Can you work these out from the model? Positions are in its coordinate system, mm. Face numbers are marked on the shaded views. A direction names the side the tool comes from. Give positions to 0.01 mm unless a question says otherwise; leave off trailing zeros. Loops run counter-clockwise (first coordinate to the right, second up) from the corner with the lowest first, then second, coordinate; pieces in that order, holes last. Notation, with made-up numbers: (84, 81.5) -> (139, 81.5) arc R32 ccw to (139, 107.5) -> close; hole circle Ø7 at (1.25, 34). An arc over 180 degrees is marked (long way). One line per question, with ' | ' between items.
from build123d import *

# Parameters (mm, degrees)
F0_R          = 12.7
F1_DEPTH      = 17.78
F2_R          = 38.1
F3_DEPTH      = 10.16
F4_R          = 12.954
F5_DEPTH      = 17.781
F5_DEPTH_BACK = 115
F6_W          = 5.08
F6_H          = 30.48
F7_DEPTH      = 38.101
F7_DEPTH_BACK = 38.101
F8_W          = 40.513
F8_H          = 5.08
F9_DEPTH      = 38.101
F9_DEPTH_BACK = 38.101
F11_DEPTH     = 6.35


# Not quite as in the source:
# - an extrude ends at something that could not be found from the text; its depth is read off the source's solid


with BuildPart() as f1:
    # F0 (on Front) → F1 (new body)
    with BuildSketch(Plane.XZ):
        Circle(F0_R)
    extrude(amount=F1_DEPTH)

    # F2 (on Front) → F3 (join)
    with BuildSketch(Plane.XZ):
        Circle(F2_R)
    extrude(amount=F3_DEPTH)

    # F4 (on Front) → F5 (cut, two sides)
    with BuildSketch(Plane.XZ) as f5_sk:
        Circle(F4_R)
    extrude(amount=F5_DEPTH, mode=Mode.SUBTRACT)
    extrude(f5_sk.sketch, amount=-F5_DEPTH_BACK, mode=Mode.SUBTRACT)

    # F6 (on Right) → F7 (cut, two sides)
    with BuildSketch(Plane.YZ) as f7_sk:
        with Locations((-2.54, 0)):
            Rectangle(F6_W, F6_H)
    extrude(amount=F7_DEPTH, mode=Mode.SUBTRACT)
    extrude(f7_sk.sketch, amount=-F7_DEPTH_BACK, mode=Mode.SUBTRACT)

    # F8 (on Top) → F9 (cut, two sides)
    with BuildSketch(Plane.XY) as f9_sk:
        with Locations((0, -2.54)):
            Rectangle(F8_W, F8_H)
    extrude(amount=-F9_DEPTH, mode=Mode.SUBTRACT)
    extrude(f9_sk.sketch, amount=F9_DEPTH_BACK, mode=Mode.SUBTRACT)

    # F10 (on face) → F11 (cut)
    with BuildSketch(Plane(origin=(0, 0, 0), x_dir=(-1, 0, 0), z_dir=(0, 1, 0))):
        with BuildLine():
            Line((1.27, -1.27), (38.0788274504, -1.27))
            ThreePointArc((38.0788274504, -1.27), (38.1, 0), (38.0788274504, 1.27))
            Line((38.0788274504, 1.27), (1.27, 1.27))
            Line((1.27, 1.27), (1.27, 38.0788274504))
            ThreePointArc((1.27, 38.0788274504), (0, 38.1), (-1.27, 38.0788274504))
            Line((-1.27, 38.0788274504), (-1.27, 1.27))
            Line((-1.27, 1.27), (-38.0788274504, 1.27))
            ThreePointArc((-38.0788274504, 1.27), (-38.1, 0), (-38.0788274504, -1.27))
            Line((-38.0788274504, -1.27), (-1.27, -1.27))
            Line((-1.27, -1.27), (-1.27, -38.0788274504))
            ThreePointArc((-1.27, -38.0788274504), (0, -38.1), (1.27, -38.0788274504))
            Line((1.27, -38.0788274504), (1.27, -1.27))
        make_face()
    extrude(amount=-F11_DEPTH, mode=Mode.SUBTRACT)


solid = f1.part
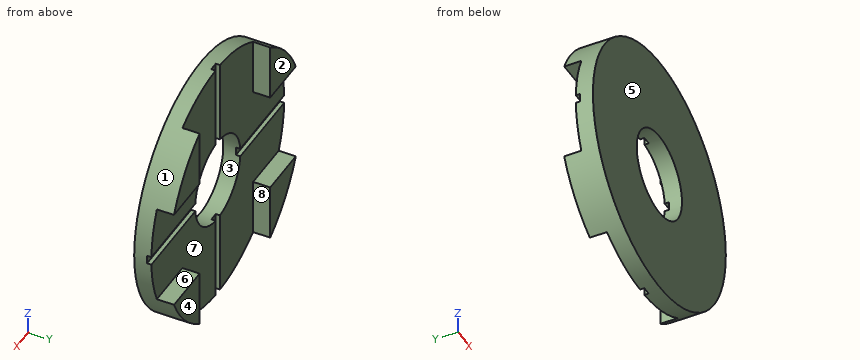
Q1. If we section it at A-A (z = 0): Write out the boundary of the cut face in (x, y).
Entries:
outline: (-38.1, -10.16) -> (-12.95, -10.16) -> (-12.95, -6.35) -> (-38.1, -6.35) -> close; (12.95, -10.16) -> (38.1, -10.16) -> (38.1, -6.35) -> (12.95, -6.35) -> close
Q2. If we section it at B-B (x = 0): Write out the boundary of the cut face in (y, z), plus the area to 3 significant figures.
Entries:
outline: (-10.16, -38.1) -> (-6.35, -38.1) -> (-6.35, -12.95) -> (-10.16, -12.95) -> close; (-10.16, 12.95) -> (-6.35, 12.95) -> (-6.35, 38.1) -> (-10.16, 38.1) -> close | area: 192 mm²
Q3. For pin 1 Ø4 at (x, y) = (20, -8) entering from -Z; pin 2 Ø2.5 at (y, z) = (-2, -23.5) entering from +X; pin 3 Ø1 at (y, z) = (-5.5, 25) entering from -X, each with a flat end and sliding along its axis, tell me the tip position at first contact or that it passes through.
Entries:
pin 1: z = -33.58 | pin 2: x = 30.93 | pin 3: x = -29.18
Q4. On a 3-axis mill with a long thin cutter (end or side, diameter ignored), from which of +Z, -Z, +X, -X, +Y, -Y can I reach the whole of each face in a straight line? I mean the marked faces 4, 5, 6, 7 and 8. Say none if no direction works.
Entries:
face 4: +Z, -Z, +X, -X, +Y | face 5: +Z, -Z, +X, -X, -Y | face 6: +X, -X, +Y | face 7: +Y | face 8: +Z, -Z, +Y
Q5. If we section it at D-D (x = 17.5): Write out the boundary of the cut face in (y, z).
Entries:
outline: (-10.16, -33.84) -> (-5.08, -33.84) -> (-5.08, -1.27) -> (-6.35, -1.27) -> (-6.35, 1.27) -> (-5.08, 1.27) -> (-5.08, 33.84) -> (-10.16, 33.84) -> close
Q6. If we mould it in two halves opening along X, with no side actions, what happens to the marked faces 1, 2 and 3? For each: pulls with the +X half, pulls with the -X half, needs draft (parallel to the pull), parting line crosses it, or undercut.
Entries:
face 1: parting line crosses it | face 2: needs draft | face 3: undercut
Q7. If I drill on probe 1 along X at (y, z) = (-7.6, 0); probe 2 along Y at (x, z) = (12.5, -24.5), over which ranges is the centre line in solid material (lowest first)? Write a range as from..to.
Entries:
probe 1: -38.1..-12.95, 12.95..38.1 | probe 2: -10.16..-5.08
Q8. If we section it at C-C (y = -8.5): Write out the boundary of the cut face in (x, z).
Entries:
outline: circle Ø76.2 at (0, 0); hole circle Ø25.91 at (0, 0)
